```python
from build123d import *

# Parameters (mm, degrees)
F0_R     = 25
F0_R_2   = 15.25
F1_DEPTH = 35
F2_R     = 10
F3_DEPTH = 200


with BuildPart() as f1:
    # F0 (on Top) → F1 (new body, symmetric)
    with BuildSketch(Plane.XY):
        Circle(F0_R)
        Circle(F0_R_2, mode=Mode.SUBTRACT)
    extrude(amount=F1_DEPTH, both=True)

    # F2 (on Right) → F3 (join)
    with BuildSketch(Plane.YZ):
        Circle(F2_R)
    extrude(amount=F3_DEPTH)


solid = f1.part
```
Geometry check sheet. Reference: the model listing, model coordinates, mm. A direction names the side the tool comes from. Give positions to 0.01 mm unless a question says otherwise; leave off trailing zeros. Order: outer loops, then holes, each group sorted by start corner. A loop starts at its lowest first (then second) coordinate and runs counter-clockwise, first axis right, second up.
1. Section check D-D, the plane x = 168.5. Enter the section's corners in (y, z).
2. Gauge pin test, flat ends, axial feed: pin 1 Ø2 at (x, z) = (137, 6) entering from -Y; pin 2 Ø8 at (y, z) = (13, 9.5) entering from -X; pin 3 Ø4 at (y, z) = (-10, 14) entering from -X. Record the tip position at first contact, or that the pin passes through.
3. Section check A-A, the plane y = 0. Enter the section's corners in (x, z).
4. Release check for a two-part mould opening along Y. For faces 3 (the face through (0, 0, 0)), 4 (the face through (-24.976, 1.099, 0.49)), 5 (the face through (-11, -11, 35)), 6 (the face through (8, -8, -6)) record: pulls with the +Y half, pulls with the -Y half, needs draft (parallel to the pull), parting line crosses it, or undercut.
5. Section check B-B, the plane z = 0. Enter the section's corners in (x, y), and give its area (3 significant figures).
6. Access from +Z, -Z, +X, -X, +Y, -Y to the whole of each face (thin tool, end or side, straight path). Record for faces 1 (the face through (-11, -11, -35)), 2 (the face through (110.22, -2.17, -9.76)).
7. Thickness scan on L1, parallel to Y at x = 0, z = -20; L2, parallel to X at y = 13, z = 11; L3, parallel to X at y = 11, z = -25.5. Record the ranges inside material, lowest first.
8. Section check C-C, the plane y = 20. Enter the section's corners in (x, z), and give its area (3 significant figures).
Values follow:
1. outline: circle Ø20 at (0, 0)
2. pin 1: stops at y = -8.66
2. pin 2: stops at x = -23.32
2. pin 3: stops at x = -23.69
3. outline: (-25, -35) - (-15.25, -35) - (-15.25, 35) - (-25, 35) - close; (0, -10) - (15.25, -10) - (15.25, -35) - (25, -35) - (25, -10) - (200, -10) - (200, 10) - (25, 10) - (25, 35) - (15.25, 35) - (15.25, 10) - (0, 10) - close
4. face 3: undercut
4. face 4: parting line crosses it
4. face 5: needs draft
4. face 6: undercut
5. outline: (22.91, -10) - (200, -10) - (200, 10) - (22.91, 10) arc R25 ccw (long way) to start; hole (0, -10) - (0, 10) - (11.51, 10) arc R15.25 ccw (long way) to (11.51, -10) - close
5. area: 5,030 mm2
6. face 1: -Z, +X, -X, +Y, -Y
6. face 2: +X
7. L1: y = -25 to -15.25, 15.25 to 25
7. L2: x = -21.35 to -7.97, 7.97 to 21.35
7. L3: x = -22.45 to -10.56, 10.56 to 22.45
8. outline: (-15, -35) - (15, -35) - (15, 35) - (-15, 35) - close
8. area: 2,100 mm2
